Input: dimensioned drawing with shaded views. Units: mm. Origin: part minimum x, y, z. Coordinates: 2 decimals unless noted, no trailing zeros. Order: outer loops, then holes, each group sorted by start corner. A loop starts at its lowest first (then second) coordinate and runs counter-clockwise, first axis right, second up. Notation, with made-up numbers: (4, -23.75) -> (12, -23.75) arc R26 cw to (12, -6.75) -> close; hole circle Ø10 at (-20.5, 73). An arc over 180 degrees is marked (long way). Answer in a Markdown table with one row per item. Add a question column.
1) Section query A-A on x = 40. Return the cut outline in (y, z).
2) Section query B-B on z = 25. Return the cut outline in (x, y).
3) Section query C-C on y = 1.2. Count the separate pieces of the cut face and the enclosed holes in it, then the cut area to 3 significant figures.
4) Ray query, line 1 (X direction, y = 1.95, z = 5); line 2 (Z direction, x = 29, y = 0.45); line 3 (X direction, y = 2.3, z = 40). Return the intervals inside material, ascending. Write a range as from..to.
5) Contact query for a flat-ended pin moving along its axis: P1, Ø1.5, axis at x = 25, z = 41.5, coming from the -Y side. Output: stop coordinate, or through.
6) Section query D-D on x = 25. Return the cut outline in (y, z), then the cut area to 3 significant figures.
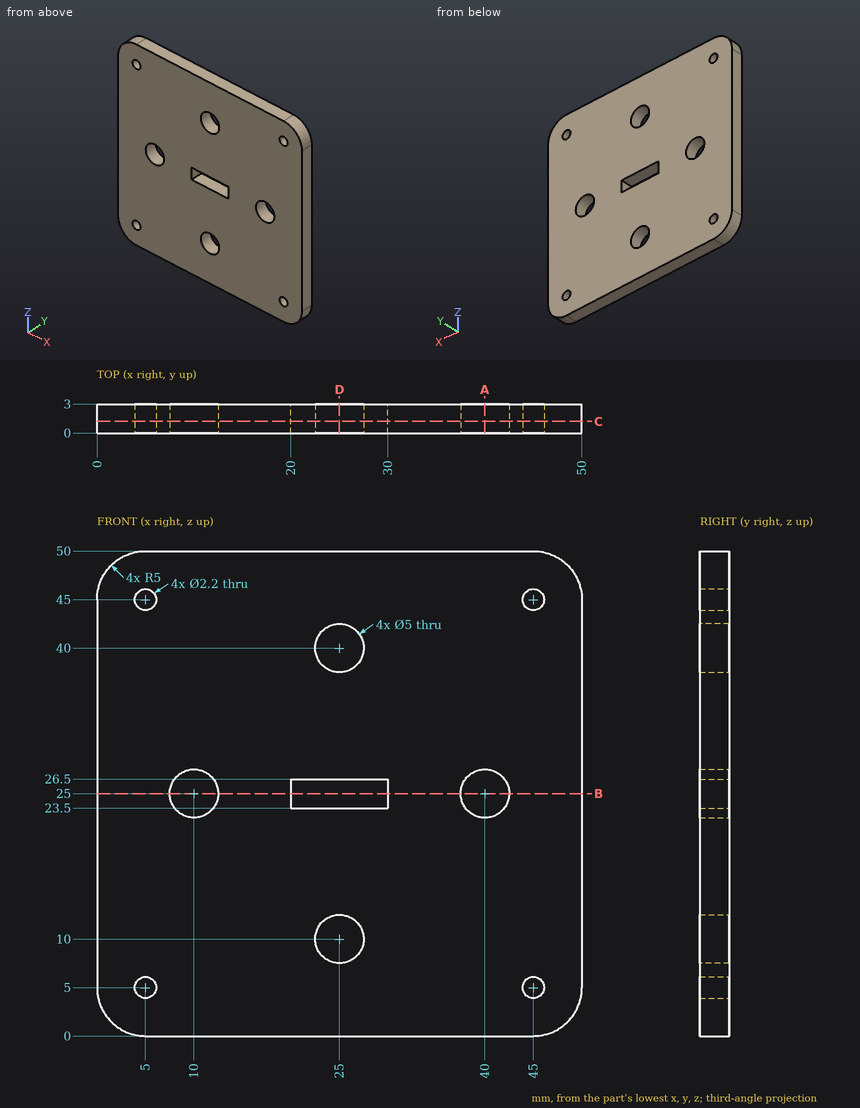
Result:
| question | item | result |
|---|---|---|
| 1 | outline | (0, 0) -> (3, 0) -> (3, 22.5) -> (0, 22.5) -> close; (0, 27.5) -> (3, 27.5) -> (3, 50) -> (0, 50) -> close |
| 2 | outline | (0, 0) -> (7.5, 0) -> (7.5, 3) -> (0, 3) -> close; (12.5, 0) -> (20, 0) -> (20, 3) -> (12.5, 3) -> close; (30, 0) -> (37.5, 0) -> (37.5, 3) -> (30, 3) -> close; (42.5, 0) -> (50, 0) -> (50, 3) -> (42.5, 3) -> close |
| 3 | separate pieces | 1 |
| 3 | enclosed holes | 9 |
| 3 | area | 2,350 mm2 |
| 4 | line 1 | 0..3.9, 6.1..43.9, 46.1..50 |
| 4 | line 2 | 0..23.5, 26.5..50 |
| 4 | line 3 | 0..22.5, 27.5..50 |
| 5 | P1 | through |
| 6 | outline | (0, 0) -> (3, 0) -> (3, 7.5) -> (0, 7.5) -> close; (0, 12.5) -> (3, 12.5) -> (3, 23.5) -> (0, 23.5) -> close; (0, 26.5) -> (3, 26.5) -> (3, 37.5) -> (0, 37.5) -> close; (0, 42.5) -> (3, 42.5) -> (3, 50) -> (0, 50) -> close |
| 6 | area | 111 mm2 |
